Geometry: final body of the model. Coordinates: model frame, mm. A direction names the side the tool comes from. Give positions to 0.01 mm unless a question says otherwise; leave off trailing zeros. Order: outer loops, then holes, each group sorted by start corner. A loop starts at its lowest first (then second) coordinate and runs counter-clockwise, first axis right, second up. Notation, with made-up numbers: (28, -5) -> (78, -5) arc R24 ccw to (78, 20) -> close; hole circle Ø5 at (7, 77.5). An arc over 180 degrees is marked (long way). Write item = value, one per line.
Autodesk Inventor part; units mm, degrees
ref_plane "YZ Plane" through (0, 0, 0) normal (1, 0, 0) x (0, 1, 0)
ref_plane "XZ Plane" through (0, 0, 0) normal (0, 1, 0) x (-1, 0, 0)
ref_plane "XY Plane" through (0, 0, 0) normal (0, 0, 1) x (1, 0, 0)
sketch "Sketch1" plane through (0, 0, 0) normal (1, 0, 0) x (0, 1, 0)
  line L0 (0, 0) -> (11.43, 0)
  line L1 (11.43, 0) -> (11.43, -19.05)
  line L2 (11.43, -19.05) -> (0, -19.05)
  line L3 (0, -19.05) -> (0, 0)
  line L4 (0, 0) -> (8.255, 0)
  line L5 (8.255, 0) -> (8.255, -15.875)
  line L6 (8.255, -15.875) -> (0, -15.875)
  line L7 (0, -15.875) -> (0, 0)
  dimension "d0" = 11.43
  dimension "d1" = 19.05
  dimension "d2" = 8.255
  dimension "d3" = 15.875
extrude "Extrusion1" add sketch "Sketch1" along normal blind 19.05 contours L0 L1 L2 L3 L6 L5
sketch "Sketch2" plane through (0, 11.43, 0) normal (0, 1, 0) x (1, 0, 0)
  line L0 (0, 19.05) -> (0, 0)
  line L1 (0, 0) -> (19.05, 0)
  line L2 (19.05, 19.05) -> (19.05, 0)
  line L3 (0, 19.05) -> (19.05, 19.05)
  point P0 (0, 0)
  point P1 (4.7625, 6.35)
  point P2 (14.2875, 6.35)
  dimension "d6" = 9.525
  dimension "d7" = 4.7625
  dimension "d8" = 19.05
  dimension "d31" = 19.05
  dimension "d34" = 6.35
  dimension "d35" = 6.35
hole "Hole1" at (4.7625, 11.43, -6.35) at (14.2875, 11.43, -6.35) direction (0, -1, 0) diameter 3.429 end through all
sketch "Sketch3" plane through (0, 0, -15.875) normal (0, 0, 1) x (1, 0, 0)
  line L0 (0, 0) -> (0, 8.255)
  line L1 (19.05, 0) -> (0, 0)
  line L2 (19.05, 8.255) -> (19.05, 0)
  line L3 (0, 8.255) -> (19.05, 8.255)
  point P0 (0, 0)
  point P1 (4.7625, 4.1275)
  point P2 (14.2875, 4.1275)
  dimension "d20" = 9.525
  dimension "d21" = 4.7625
  dimension "d22" = 4.1275
  dimension "d23" = 4.1275
  dimension "d32" = 19.05
  dimension "d33" = 8.255
hole "Hole2" at (4.7625, 4.1275, -15.875) at (14.2875, 4.1275, -15.875) direction (0, 0, -1) diameter 3.81 end through all
properties part number "TensionerPlate4a" material "ABS Plastic"
1) Section query A-A (z = -6.35). Output: boundary loops of the cut face in (x, y) (3 decimals), plus the area to 3 significant figures.
Check sheet entries:
outline = (0, 8.255) -> (3.048, 8.255) -> (3.048, 11.43) -> (0, 11.43) -> close; (6.477, 8.255) -> (12.573, 8.255) -> (12.573, 11.43) -> (6.477, 11.43) -> close; (16.002, 8.255) -> (19.05, 8.255) -> (19.05, 11.43) -> (16.002, 11.43) -> close
area = 38.7 mm²
2) Section query C-C (x = 8.75). Output: boundary loops of the cut face in (y, z) (3 decimals), plus the area to 3 significant figures.
Check sheet entries:
outline = (0, -19.05) -> (11.43, -19.05) -> (11.43, 0) -> (8.255, 0) -> (8.255, -15.875) -> (0, -15.875) -> close
area = 86.7 mm²
3) Reachability of faces 4 (the face through (9, 4, -15.875)), 5 (the face through (0, 9, -12)) from +Z, -Z, +X, -X, +Y, -Y: full face, straight path, thin tool, end or side. Return the list, or none.
Check sheet entries:
face_4 = +Z, +X, -X, -Y
face_5 = +Z, -Z, -X, +Y, -Y
4) Section query B-B (y = 3.75). Output: boundary loops of the cut face in (x, z) (3 decimals), plus the area to 3 significant figures.
Check sheet entries:
outline = (0, -19.05) -> (2.895, -19.05) -> (2.895, -15.875) -> (0, -15.875) -> close; (6.63, -19.05) -> (12.42, -19.05) -> (12.42, -15.875) -> (6.63, -15.875) -> close; (16.155, -19.05) -> (19.05, -19.05) -> (19.05, -15.875) -> (16.155, -15.875) -> close
area = 36.8 mm²
5) Mould query, pull axis X, two halves, no side actions, for faces 1 (the face through (12.84, 9.82, -5.43)), 2 (the face through (19.05, 9, -12)), 3 (the face through (9, 0, -17)). Classes: +X half, -X half, draft (parallel to the pull), parting line (faces both ways), or undercut.
Check sheet entries:
face_1 = undercut
face_2 = +X half
face_3 = draft
6) First-contact query: P1, Ø6, axis at x = 13.5, z = -7, coming from the -Y side (3 decimals). Flat tip, straight axial feed; report the tip coordinate or a pass-through.
Check sheet entries:
P1 = 8.255
7) Line query: line 1 (X direction, y = 8.95, z = -6.35); line 2 (X direction, y = 3.25, z = -16); line 3 (Z direction, x = 18.25, y = 1) (3 decimals). Output: solid intervals per line, ascending. Write a range as from..to.
Check sheet entries:
line_1 = 0..3.05, 6.48..12.57, 16..19.05
line_2 = 0..3.07, 6.45..12.6, 15.98..19.05
line_3 = -19.05..-15.875
8) Section query D-D (y = 8). Output: boundary loops of the cut face in (x, z) (3 decimals).
Check sheet entries:
outline = (0, -19.05) -> (19.05, -19.05) -> (19.05, -15.875) -> (0, -15.875) -> close
